Design review of the part built by this model. Coordinates are the model's own, in mm. Face numbers are marked on the shaded views. A direction names the side the tool comes from. Give positions to 0.01 mm unless a question says otherwise; leave off trailing zeros. Write each loop counter-clockwise with the first axis right and the second up, starting at its lowest first coordinate (ties: lowest second). Pieces come first, ordered by that corner, then holes. Notation, with made-up numbers: M 61.25,85.5 L 98.25,85.5 A16 cw 98.25,99.5 Z; hole C 35,22.5 d11. An arc over 180 degrees is marked long. One line per item, written item: value. Start each with the question number.
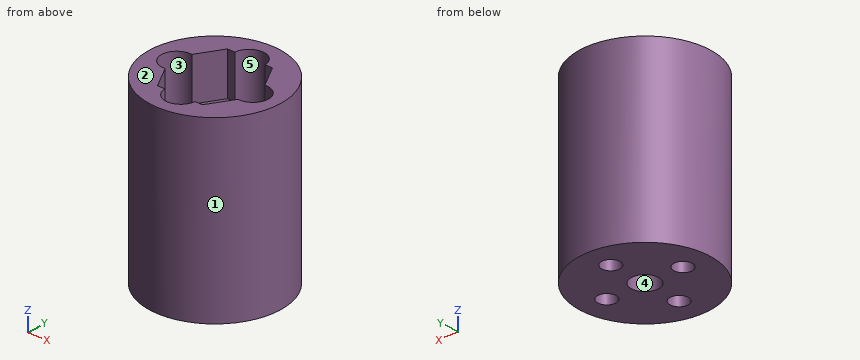
Autodesk Inventor part; units mm, degrees
ref_plane "Work Plane2" through (0, 0, 5) normal (0, 0, -1) x (-1, 0, 0)
ref_plane "YZ Plane" through (0, 0, 0) normal (1, 0, 0) x (0, 1, 0)
ref_plane "XZ Plane" through (0, 0, 0) normal (0, 1, 0) x (-1, 0, 0)
sketch "Sketch1" plane through (0, 0, 0) normal (0, 0, 1) x (1, 0, 0)
  circle A0 centre (0, 0) radius 10.75
  circle A1 centre (0, 0) radius 2.25
  dimension "d0" = 21.5
  dimension "d1" = 4.5
extrude "Extrusion1" add sketch "Sketch1" along normal blind 29
sketch "Sketch2" plane through (0, 0, 29) normal (0, 0, 1) x (1, 0, 0)
  line L0 (7.5, 0) -> (3.75, -6.4952)
  line L1 (3.75, -6.4952) -> (-3.75, -6.4952)
  line L2 (-3.75, -6.4952) -> (-7.5, 0)
  line L3 (-7.5, 0) -> (-3.75, 6.4952)
  line L4 (-3.75, 6.4952) -> (3.75, 6.4952)
  line L5 (3.75, 6.4952) -> (7.5, 0)
  point P0 (0, 0)
  point P1 (0, 0)
  dimension "d4" = 15
extrude "Extrusion2" cut sketch "Sketch2" against normal blind 7
sketch "Sketch9" plane through (0, 0, 29) normal (0, 0, 1) x (1, 0, 0)
  circle A0 centre (0, -6.35) radius 1.5
  circle A1 centre (0, 6.35) radius 1.5
  line L0 (0, 6.35) -> (0, -6.35) construction
  circle A2 centre (6.35, 0) radius 1.5
  circle A3 centre (-6.35, 0) radius 1.5
  line L1 (-6.35, 0) -> (6.35, 0) construction
  point P0 (0, 0)
  point P1 (0, 0)
  dimension "d19" = 3
  dimension "d20" = 3
  dimension "d21" = 12.7
  dimension "d22" = 3
  dimension "d23" = 3
  dimension "d24" = 12.7
extrude "Extrusion6" cut sketch "Sketch9" against normal through all
ref_plane "Work Plane2" through (0, 0, 5) normal (0, 0, -1) x (-1, 0, 0)
sketch "Sketch11" plane through (0, 0, 5) normal (0, 0, -1) x (-1, 0, 0)
  circle A0 centre (-6.35, 0) radius 1.5
  spline S0 degree 2 poles (-1.5, 6.35) (-1.5, 8.9481) (0.75, 7.649) (3, 6.35) (0.75, 5.051) (-1.5, 3.7519) (-1.5, 6.35) knots 0 0 0 0.333333 0.333333 0.666667 0.666667 1 1 1 weights 1 0.5 1 0.5 1 0.5 1
  circle A1 centre (6.35, 0) radius 1.5
  circle A2 centre (-6.35, 0) radius 2.5
  circle A3 centre (0, 6.35) radius 1.5
  circle A4 centre (0, 6.35) radius 2.5
  circle A5 centre (6.35, 0) radius 2.5
  circle A6 centre (0, -6.35) radius 1.5
  circle A7 centre (0, -6.35) radius 2.5
  point P0 (0, 0)
  dimension "d32" = 5
  dimension "d33" = 5
  dimension "d34" = 5
  dimension "d35" = 5
extrude "Extrusion7" cut sketch "Sketch11" against normal through all contours A0 | S0 | A1 | A2 | A4 | A5 | A6 | A7
properties part number "AA032" material "ABS Plastic"
Q1. Take a section at D-D, the plane y = -5.25. Give the boundary of the cut face in (x, z) (3 decimals), then the cut area to 3 significant figures.
Q2. For P1, Ø1.5, axis at x = -6, z = 8, coming from the +Y side; P2, Ø1.5, axis at x = 5, y = 0, coming from the +Z side; P3, Ø4, axis at y = 8.5, z = 5.5, coming from the +X side, all flat-tipped, find the tip position at first contact; note any pin that passes through.
Q3. Take a section at A-A, the plane y = 0. Give the boundary of the cut face in (x, z), then the cut area to 3 significant figures.
Q4. The part is to be moulded in two halves that separate along X. For the marked faces 1, 2 and 3, say which applies: pulls with the +X half, pulls with the -X half, needs draft (parallel to the pull), parting line crosses it, or undercut.
Q5. Wall thickness on line 1 (Y direction, x = 0, z = 21); line 2 (Y direction, x = 1, z = 16); line 3 (Y direction, x = -6.5, z = 6): over which ranges is each line inside the solid? List them lowest first. Write a range as from..to.
Q6. Take a section at C-C, the plane z = 15.5. Give the boundary of the cut face in (x, y).
Q7. Machinability: for the marked faces 4 and 5, which of the approach directions +Z, -Z, +X, -X, +Y, -Y give a long, thin tool a straight path to every point of the face, cutting with its end or side? Answer none if there is none.
Results list:
1. outline: M -9.381,0 L -1.02,0 L -1.02,5 L -2.245,5 L -2.245,22 L -4.469,22 L -4.469,29 L -9.381,29 Z; M 1.02,0 L 9.381,0 L 9.381,29 L 4.469,29 L 4.469,22 L 2.245,22 L 2.245,5 L 1.02,5 Z
1. area: 395 mm^2
2. P1: stops at y = 9.38
2. P2: stops at z = 5
2. P3: stops at x = 8.56
3. outline: M -10.75,0 L -7.85,0 L -7.85,5 L -8.85,5 L -8.85,29 L -10.75,29 Z; M -4.85,0 L -2.25,0 L -2.25,22 L -3.85,22 L -3.85,5 L -4.85,5 Z; M 2.25,0 L 4.85,0 L 4.85,5 L 3.85,5 L 3.85,22 L 2.25,22 Z; M 7.85,0 L 10.75,0 L 10.75,29 L 8.85,29 L 8.85,5 L 7.85,5 Z
3. area: 201 mm^2
4. face 1: parting line crosses it
4. face 2: needs draft
4. face 3: undercut
5. line 1: y = -10.75..-8.85, -3.85..-2.25, 2.25..3.85, 8.85..10.75
5. line 2: y = -10.7..-8.64, -4.06..-2.02, 2.02..4.06, 8.64..10.7
5. line 3: y = -8.56..-2.5, 2.5..8.56
6. outline: C 0,0 d21.5; hole C -6.35,0 d5; hole C 0,-6.35 d5; hole C 0,6.35 d5; hole C 0,0 d4.5; hole C 6.35,0 d5
7. face 4: +Z, -Z
7. face 5: +Z
